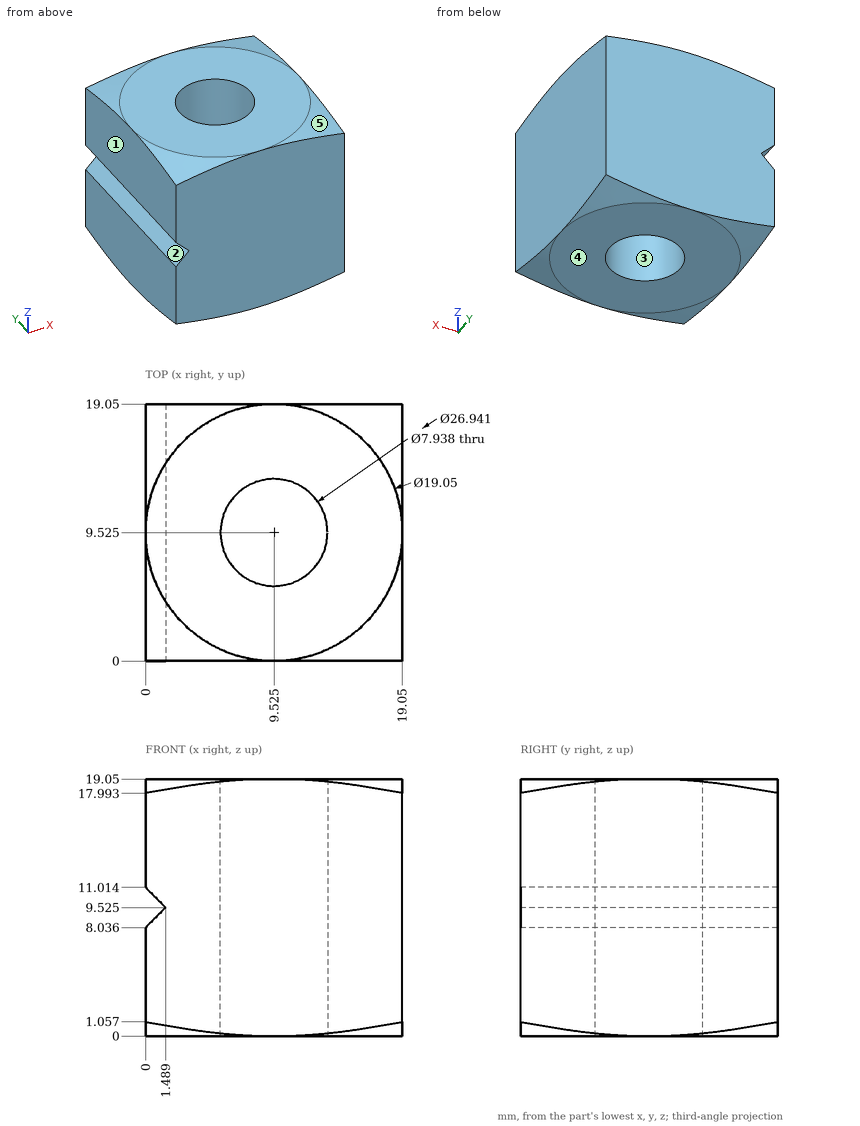
Answer from the drawing. Dimensions are ordinates in mm from the lowest x, y and z of the part. A direction names the side the tool comes from. Coordinates: 2 decimals unless noted, no trailing zeros.
Q1. This flat-tipped pin is pushed along its axis until it touches: pin 1 Ø4 at (x, y) = (15.5, 15.5) entering from -Z. Where does it stop, or does it pass through?
Q2. The mould has two halves that part along Y. Classify the marked faces 3, 4 and 5: +Y half, -Y half, draft (parallel to the pull), parting line (faces both ways), or undercut.
Q3. Which of the six approach directions +Z, -Z, +X, -X, +Y, -Y give full straight-line access (tool end or side, diameter ignored) to the marked faces 1 and 2?
Q4. Consider probe 1 along Y at (x, z) = (11, 9.25); probe 2 along X at (y, z) = (7.5, 14.5); probe 3 along Z at (x, y) = (17.5, 3.75) (1 decimal). Determine where each line is inside the solid, lowest interval first.
Results below:
1. pin 1: stops at z = 0
2. face 3: undercut
2. face 4: draft
2. face 5: -Y half
3. face 1: +Z, -Z, -X, +Y, -Y
3. face 2: -X, +Y, -Y
4. probe 1: y = 0 to 5.84, 13.21 to 19.05
4. probe 2: x = 0 to 6.11, 12.94 to 19.05
4. probe 3: z = 0.1 to 19
